The drawing under review shows one solid part. Ordinate dimensions are in mm from its lowest x, y, z. Coordinates: 2 decimals unless noted, no trailing zeros. Loops run counter-clockwise (first coordinate to the right, second up) from the corner with the lowest first, then second, coordinate; pieces in that order, holes last.
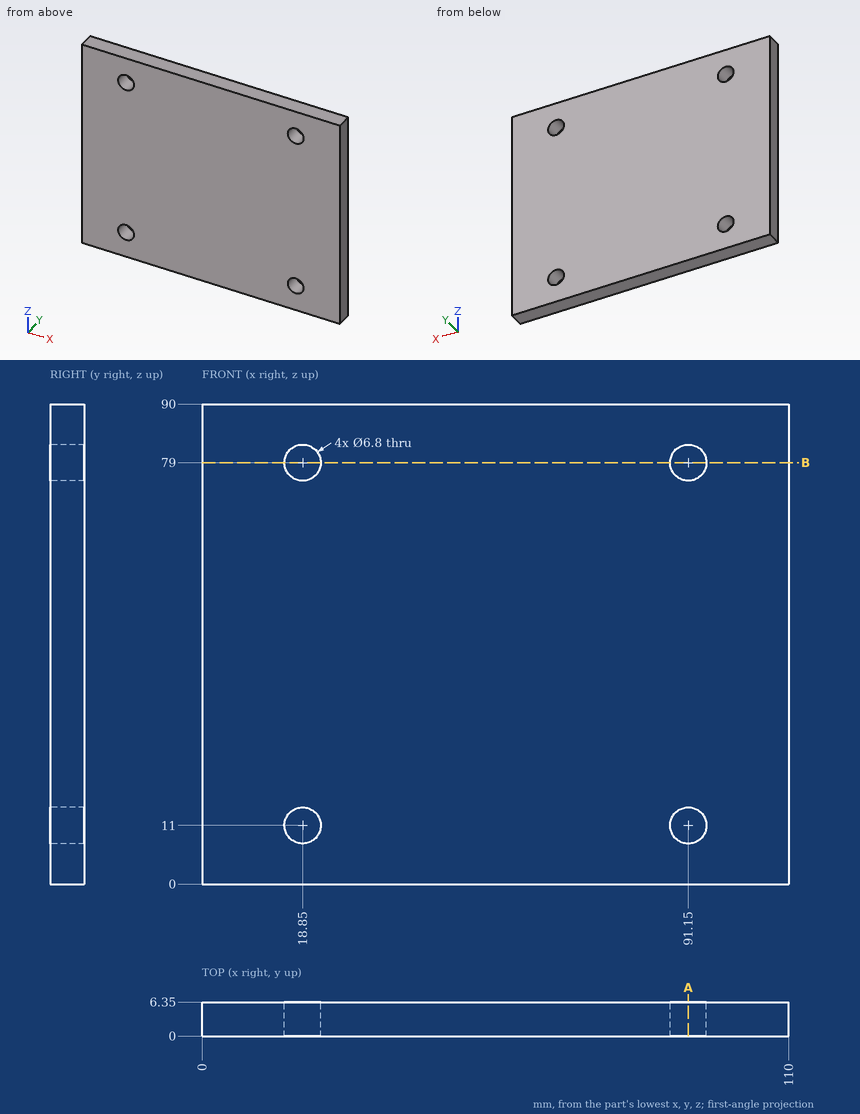
Q1. Take a section at B-B, the plane z = 79. Write out the cut boundary in (x, y), then the cut area to 3 significant figures.
Q2. Clearance check with a flat-ended pin moving along its axis: pin 1 Ø4 at (x, z) = (91.15, 79) entering from -Y. State where the tip first meets the part, or that it passes through.
Q3. For line 1 (X direction, y = 4, z = 11); line 2 (Z direction, x = 89.5, y = 6); line 3 (Z direction, x = 89, y = 2.75), list the stretches that pass through material, from the lowest coordinate up.
Q4. Take a section at A-A, the plane x = 91.15. Write out the cut boundary in (y, z), then the cut area to 3 significant figures.
Entries:
1. outline: (0, 0) - (15.45, 0) - (15.45, 6.35) - (0, 6.35) - close; (22.25, 0) - (87.75, 0) - (87.75, 6.35) - (22.25, 6.35) - close; (94.55, 0) - (110, 0) - (110, 6.35) - (94.55, 6.35) - close
1. area: 612 mm2
2. pin 1: passes through
3. line 1: x = 0 to 15.45, 22.25 to 87.75, 94.55 to 110
3. line 2: z = 0 to 8.03, 13.97 to 76.03, 81.97 to 90
3. line 3: z = 0 to 8.37, 13.63 to 76.37, 81.63 to 90
4. outline: (0, 0) - (6.35, 0) - (6.35, 7.6) - (0, 7.6) - close; (0, 14.4) - (6.35, 14.4) - (6.35, 75.6) - (0, 75.6) - close; (0, 82.4) - (6.35, 82.4) - (6.35, 90) - (0, 90) - close
4. area: 485 mm2
